Model file for the job. Use its own axes, mm. A direction names the side the tool comes from. Coordinates: 2 decimals unless noted, no trailing zeros. Write each loop counter-clockwise with the first axis right and the second up, starting at its lowest first coordinate (ties: lowest second). Pieces come first, ordered by that corner, then holes.
Q1. Band-saw the part on D-D, the plane x = -20.5. Write the cut outline in (y, z), plus the area to 3 significant figures.
Q2. Band-saw the part on C-C, the plane z = 8. Write the cut outline in (x, y) (3 decimals), plus the area to 3 significant figures.
Q3. Band-saw the part on A-A, the plane y = 1.5. Write the cut outline in (x, z).
Q4. Band-saw the part on B-B, the plane z = 29. Write the cut outline in (x, y) (3 decimals), plus the area to 3 significant figures.
Q5. Pin check, flat tips, straight feed: P1, Ø3, axis at x = 11.5, z = 40, coming from the -Y side; P2, Ø1.5, axis at y = 6, z = 61.5, coming from the +X side; P3, Ø12, axis at x = 10.5, z = 55.5, coming from the -Y side. Stop position of each tip, or through.
Q6. Which spindle directions (+Z, -Z, +X, -X, +Y, -Y) get a long thin tool onto all of the face, cutting with end or side? Do faces 1 (the flat face through (-0.75, 26, 25)), 2 (the flat face through (5, 12, 0)), 3 (the flat face through (-22.4, -13.8, 24.5)). Say none if no direction does.
Q7. Pull direction X, two halves, no side cores. Call faces 4 (the flat face through (0.23, 24.52, 47.47)), 5 (the flat face through (0.75, 26, 25)), 6 (the flat face through (22.166, -13.663, 24.544)): released by +X, released by -X, zero draft, split by the parting line, or undercut.
Q8. Drill centre lines: probe 1 along X at (y, z) = (-11, 16.5); probe 2 along Y at (x, z) = (0, 21.5); probe 3 along X at (y, z) = (11, 11.5). Where is each one in solid material? Low to high.
from build123d import *

# Parameters (mm, degrees)
F0_R     = 12.7
F1_DEPTH = 75
F3_DEPTH = 1.5
F4_R     = 5
F6_COUNT = 3
F6_ANGLE = 240


# Not quite as in the source:
# - a feature names something its author has since deleted; it is built from what else it names


with BuildPart() as f1:
    # F0 (on Top) → F1 (new body)
    with BuildSketch(Plane.XY):
        with BuildLine():
            ThreePointArc((-0.75, 13.9298241195), (-9.595311355, -10.125833299), (13.95, 0))
            ThreePointArc((13.95, 0), (10.125833299, 9.595311355), (0.75, 13.9298241195))
            ThreePointArc((0.75, 13.9298241195), (0, 13.95), (-0.75, 13.9298241195))
        make_face()
        Circle(F0_R, mode=Mode.SUBTRACT)
        with BuildLine():
            ThreePointArc((-0.75, 13.9298241195), (0, 13.95), (0.75, 13.9298241195))
            Line((0.75, 13.9298241195), (0.75, 38.9298241195))
            Line((0.75, 38.9298241195), (0, 38.9298241195))
            Line((0, 38.9298241195), (-0.75, 38.9298241195))
            Line((-0.75, 38.9298241195), (-0.75, 13.9298241195))
        make_face()
    extrude(amount=F1_DEPTH)

    # F2 (on face) → F3 (cut, through all)
    with BuildSketch(Plane.YZ.offset(0.75)):
        Polygon((38.9298241195, 75), (13.9298241195, 75), (38.9298241195, 10), align=None)
    extrude(amount=-F3_DEPTH, mode=Mode.SUBTRACT)

    # F4 (call 1 of 2: OpenCascade refuses the feature's edges together)
    f4_edges = [f1.edges().sort_by_distance(p)[0] for p in [
        (0.75, 13.929824, 37.5),
    ]]
    fillet(f4_edges, radius=F4_R)

    # F4#2 (call 2 of 2)
    f4_2_edges = [f1.edges().sort_by_distance(p)[0] for p in [
        (-0.75, 13.929824, 37.5),
    ]]
    fillet(f4_2_edges, radius=F4_R)

    # F6: F1 ×3 about axis
    f6_axis = Axis((0, 0, 42.7156351507), (0, 0, 1))


with BuildPart() as f1_1:
    add(f1.part)
    for i in range(1, F6_COUNT):
        add(f1.part.rotate(f6_axis, i * F6_ANGLE / (F6_COUNT - 1)))


solid = f1_1.part
Answer sheet:
1. outline: (-12.7, 0) - (-10.97, 0) - (-10.97, 50.8) - (-12.7, 48.55) - close
1. area: 86.0 mm2
2. outline: (-34.089, -18.815) - (-33.339, -20.114) - (-15.262, -9.678) arc R5 cw to (-9.395, -10.312) arc R13.95 ccw to (9.395, -10.312) arc R5 cw to (15.262, -9.678) - (33.339, -20.114) - (34.089, -18.815) - (16.012, -8.379) arc R5 cw to (13.628, -2.98) arc R13.95 ccw to (4.233, 13.292) arc R5 cw to (0.75, 18.057) - (0.75, 38.93) - (-0.75, 38.93) - (-0.75, 18.057) arc R5 cw to (-4.233, 13.292) arc R13.95 ccw to (-13.628, -2.98) arc R5 cw to (-16.012, -8.379) - close; hole circle Ø25.4 at (0, 0)
2. area: 235 mm2
3. outline: (-13.87, 0) - (-12.61, 0) - (-12.61, 75) - (-13.87, 75) - close; (12.61, 0) - (13.87, 0) - (13.87, 75) - (12.61, 75) - close
4. outline: (-27.761, -15.162) - (-27.011, -16.461) - (-15.262, -9.678) arc R5 cw to (-9.395, -10.312) arc R13.95 ccw to (9.395, -10.312) arc R5 cw to (15.262, -9.678) - (27.011, -16.461) - (27.761, -15.162) - (16.012, -8.379) arc R5 cw to (13.628, -2.98) arc R13.95 ccw to (4.233, 13.292) arc R5 cw to (0.75, 18.057) - (0.75, 31.622) - (-0.75, 31.622) - (-0.75, 18.057) arc R5 cw to (-4.233, 13.292) arc R13.95 ccw to (-13.628, -2.98) arc R5 cw to (-16.012, -8.379) - close; hole circle Ø25.4 at (0, 0)
4. area: 203 mm2
5. P1: stops at y = -9.84
5. P2: stops at x = 12.92
5. P3: stops at y = -13.2
6. face 1: +Z, -Z, -X, +Y
6. face 2: -Z, +X, -X, +Y, -Y
6. face 3: +Z, -Z, -Y
7. face 4: zero draft
7. face 5: released by +X
7. face 6: undercut
8. probe 1: x = -20.55 to -17.55, -8.58 to -6.35, 6.35 to 8.58, 17.55 to 20.55
8. probe 2: y = -13.95 to -12.7, 12.7 to 34.51
8. probe 3: x = -8.58 to -6.35, 6.35 to 8.58
